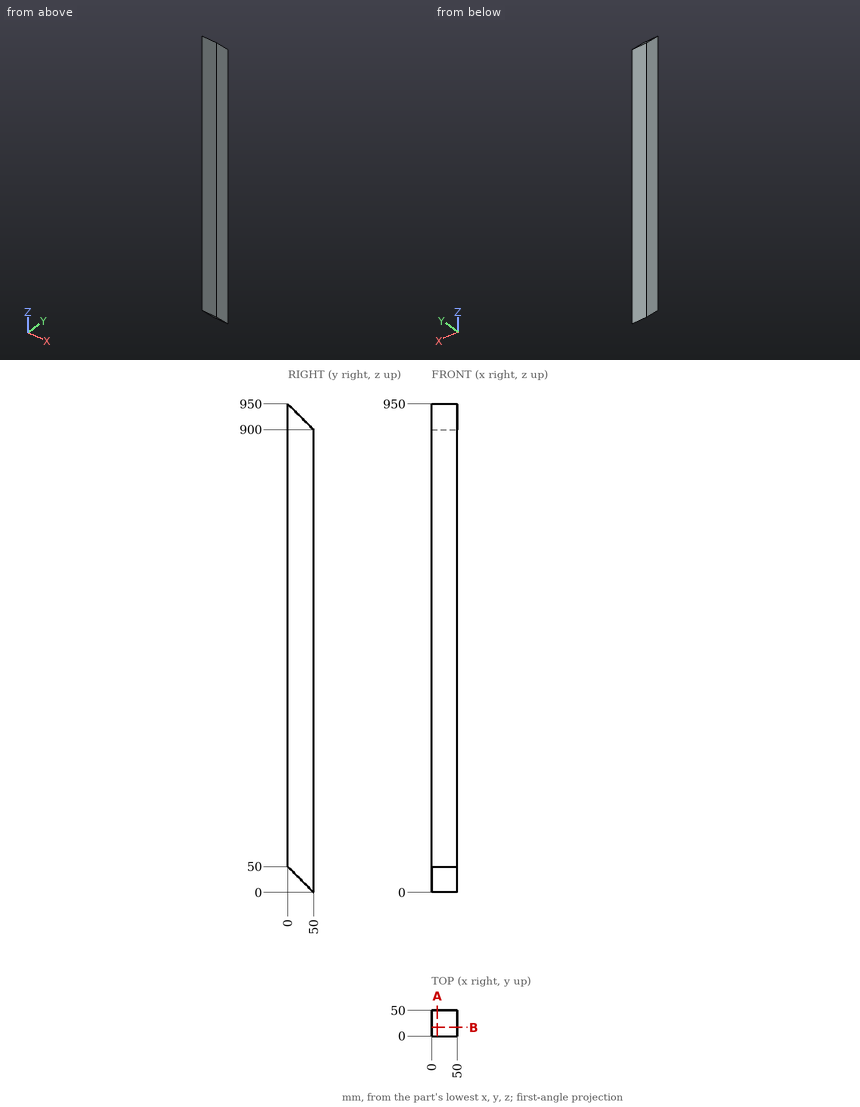
Here's the drawing with two shaded views (mm, measured from the low corner). I have some questions. Give positions to 0.01 mm unless a question says otherwise; leave off trailing zeros. Order: outer loops, then holes, each group sorted by start corner. A loop starts at its lowest first (then second) coordinate and runs counter-clockwise, first axis right, second up. Notation, with made-up numbers: M 52,64 L 83,64 A25 cw 83,79 Z; hole C 65.25,-33 d10. An arc over 180 degrees is marked long. One line per item, written item: value.
1) I want a section at B-B, the plane y = 17. List the corners of the cut face in (x, z) for me, plus the area to 3 significant figures.
Answer sheet:
outline: M 0,33 L 50,33 L 50,933 L 0,933 Z
area: 45,000 mm^2
2) For P1, Ø2, axis at x = 23.5, y = 17.5, coming from the +Z side; P2, Ø2, axis at x = 40, y = 13, coming from the +Z side, each with a flat end and sliding along its axis, tell me the tip position at first contact or that it passes through.
Answer sheet:
P1: stops at z = 933.5
P2: stops at z = 938
3) Please list where these lines run through material, in increasing order: line 1 along Z through (x, y) = (11.5, 12.5); line 2 along Z through (x, y) = (2.5, 36.5).
Answer sheet:
line 1: z = 37.5 to 937.5
line 2: z = 13.5 to 913.5
4) I want a section at A-A, the plane x = 11.5. List the corners of the cut face in (y, z) for me, plus the area to 3 significant figures.
Answer sheet:
outline: M 0,50 L 50,0 L 50,900 L 0,950 Z
area: 45,000 mm^2
